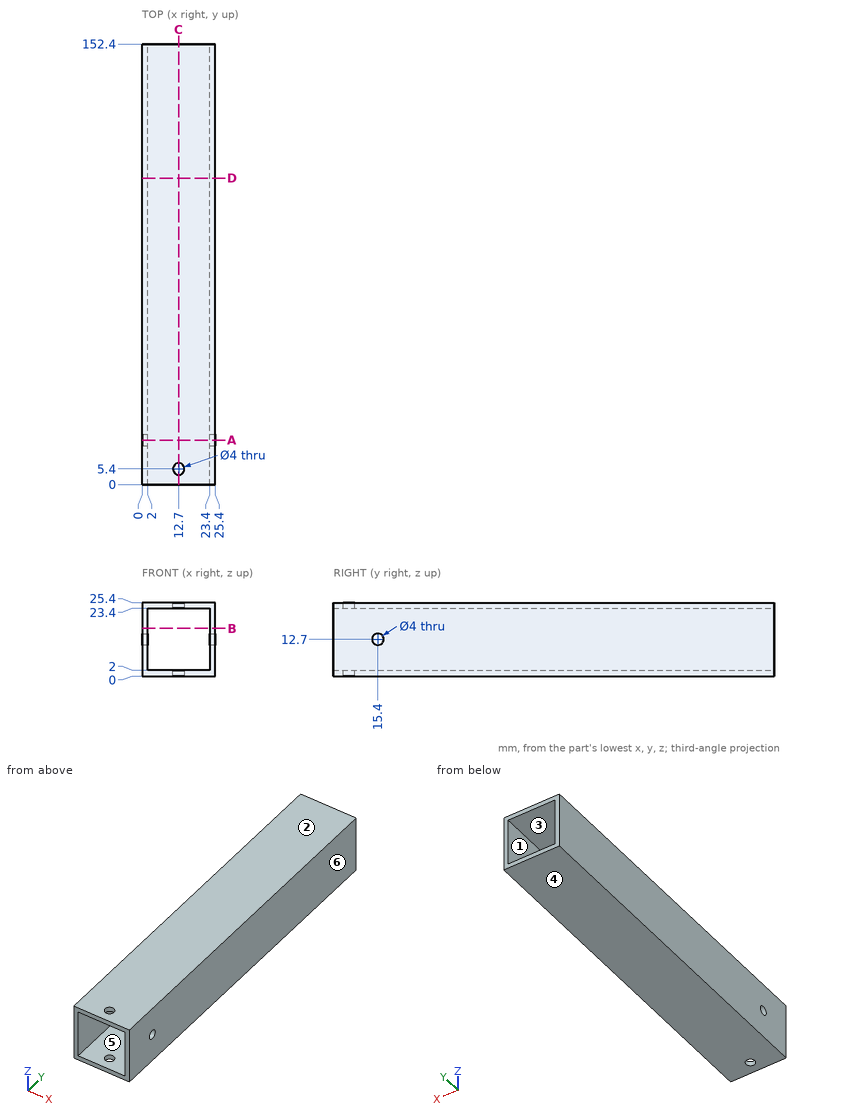
The figure shows three views and two pictorial views of one solid part (mm, origin at its lowest corner). Answer the questions. A direction names the side the tool comes from. Give positions to 0.01 mm unless a question says otherwise; leave off trailing zeros. Write each loop counter-clockwise with the first axis right and the second up, starting at its lowest first coordinate (ties: lowest second). Pieces come first, ordered by that corner, then holes. Notation, with made-up numbers: (16.25, 41) - (74.25, 41) arc R9 cw to (74.25, 52) - close; hole circle Ø6 at (22.5, 28). An arc over 180 degrees is marked (long way). Use one line per item in the form item = value.
1. A cutting plane is placed at B-B (z = 16.5). Write down the section's boundary in (x, y), and give its area (3 significant figures).
Filled in:
outline = (0, 0) - (2, 0) - (2, 152.4) - (0, 152.4) - close; (23.4, 0) - (25.4, 0) - (25.4, 152.4) - (23.4, 152.4) - close
area = 610 mm^2
2. Consider L1, parallel to Z at x = 10, y = 65.5; L2, parallel to Y at x = 12.7, z = 24.9. Determine where each line is inside the solid, lowest interval first.
Filled in:
L1 = 0 to 2, 23.4 to 25.4
L2 = 0 to 3.4, 7.4 to 152.4
3. This flat-tipped pin is pushed along its axis until it touches: pin 1 Ø5 at (x, y) = (12.7, 5.4) entering from +Z. Where does it stop, or does it pass through?
Filled in:
pin_1 = 25.4
4. Determine the mould class of the marked faces 3, 4, 5 and 6 for opening direction X: released by +X, released by -X, zero draft, split by the parting line, or undercut.
Filled in:
face_3 = undercut
face_4 = zero draft
face_5 = undercut
face_6 = released by +X
5. For the marked faces 1 and 2, determine the directions among +Z, -Z, +X, -X, +Y, -Y from which every point of the face is accessible in a straight line to the end or side of a thin tool.
Filled in:
face_1 = +Y, -Y
face_2 = +Z, +X, -X, +Y, -Y
6. A cutting plane is placed at C-C (x = 12.7). Write down the section's boundary in (y, z), and give its area (3 significant figures).
Filled in:
outline = (0, 0) - (3.4, 0) - (3.4, 2) - (0, 2) - close; (0, 23.4) - (3.4, 23.4) - (3.4, 25.4) - (0, 25.4) - close; (7.4, 0) - (152.4, 0) - (152.4, 2) - (7.4, 2) - close; (7.4, 23.4) - (152.4, 23.4) - (152.4, 25.4) - (7.4, 25.4) - close
area = 594 mm^2
7. A cutting plane is placed at A-A (y = 15.4). Write down the section's boundary in (x, z), and give its area (3 significant figures).
Filled in:
outline = (0, 0) - (25.4, 0) - (25.4, 10.7) - (23.4, 10.7) - (23.4, 2) - (2, 2) - (2, 10.7) - (0, 10.7) - close; (0, 14.7) - (2, 14.7) - (2, 23.4) - (23.4, 23.4) - (23.4, 14.7) - (25.4, 14.7) - (25.4, 25.4) - (0, 25.4) - close
area = 171 mm^2
8. A cutting plane is placed at D-D (y = 106). Write down the section's boundary in (x, z).
Filled in:
outline = (0, 0) - (25.4, 0) - (25.4, 25.4) - (0, 25.4) - close; hole (2, 2) - (23.4, 2) - (23.4, 23.4) - (2, 23.4) - close
